Input: part model. Units: mm. Frame: model coordinates. A direction names the side the tool comes from. Round coordinates to 2 decimals unless told otherwise and drop trailing zeros. Write each loop counter-clockwise with the first axis right and the second up, starting at its lowest first coordinate (ties: lowest second). Pieces come first, ordered by that corner, then holes. Notation, with made-up numbers: M -21,14.25 L -3,14.25 A20 cw -3,41.25 Z; hole C -16,84.5 d11. An arc over 180 degrees is marked long. Write each question's results on one line, items separated by ' | '. Start each with the question number.
Autodesk Inventor part; units mm, degrees
ref_plane "YZ Plane" through (0, 0, 0) normal (1, 0, 0) x (0, 1, 0)
ref_plane "XZ Plane" through (0, 0, 0) normal (0, 1, 0) x (-1, 0, 0)
ref_plane "XY Plane" through (0, 0, 0) normal (0, 0, 1) x (1, 0, 0)
sketch "Sketch1" plane through (0, 0, 0) normal (0, 0, 1) x (1, 0, 0)
  line L0 (0, 0) -> (0, 69)
  line L1 (0, 69) -> (70, 69)
  line L2 (70, 69) -> (70, 0)
  line L3 (70, 0) -> (0, 0)
  dimension "d0" = 69
  dimension "d1" = 70
extrude "Extrusion1" add sketch "Sketch1" along normal blind 56
sketch "Sketch2" plane through (0, 0, 56) normal (0, 0, 1) x (1, 0, 0)
  line L0 (0, 0) -> (37, 0)
  line L1 (37, 0) -> (37, 47)
  line L2 (37, 47) -> (0, 47)
  line L3 (0, 47) -> (0, 0)
  dimension "d4" = 37
  dimension "d5" = 47
emboss "Emboss1" sketch "Sketch2" operation cut depth 29 direction (0, 0, -1)
sketch "Sketch3" plane through (0, 0, 56) normal (0, 0, 1) x (1, 0, 0)
  circle A0 centre (62, 61) radius 3
  point P0 (0, 0)
  point P1 (70, 69)
  dimension "d10" = 6
hole "Hole1" at (62, 61, 56) direction (0, 0, -1) diameter 6 end through all
sketch "Sketch4" plane through (0, 0, 0) normal (-1, 0, 0) x (0, 0, 1)
  circle A0 centre (8, 50) radius 3
  point P0 (0, 69)
  dimension "d20" = 6
hole "Hole2" at (0, 50, 8) direction (1, 0, 0) diameter 6 end through all
sketch "Sketch5" plane through (0, 69, 0) normal (0, 1, 0) x (1, 0, 0)
  circle A0 centre (51.2959, -19) radius 3
  dimension "d30" = 6
hole "Hole3" at (51.2959, 69, 19) direction (0, -1, 0) diameter 6 end through all
sketch "Sketch6" plane through (0, 47, 27) normal (0, 0, 1) x (1, 0, 0)
  circle A0 centre (14.5, -32.5) radius 9.5
  dimension "d40" = 19
hole "Hole4" at (14.5, 14.5, 27) direction (0, 0, -1) diameter 19 depth 6
sketch "Sketch7" plane through (37, 0, 56) normal (-1, 0, 0) x (0, 0, 1)
  circle A0 centre (-14.5, 32.5) radius 9.5
  point P0 (-56, 0)
  point P1 (-29, 47)
  dimension "d50" = 19
hole "Hole5" at (37, 32.5, 41.5) direction (1, 0, 0) diameter 19 depth 6
properties part number "Tophjørne1" material "PC/ABS Plastic"
1. Draft query along X for faces 1 (the face through (54.225, 34.017, 18.35)), 2 (the face through (43, 32, 41)), 3 (the face through (11.646, 5.439, 23.958)), 4 (the face through (18, 24, 27)). Return one class per face: +X half, -X half, draft (parallel to the pull), parting line (faces both ways), or undercut.
2. Cut plane D-D on y = 33.5. Output: boundary loops of the cut face in (x, z), and give its area (3 significant figures).
3. Line query: L1, parallel to X at y = 19, z = 19; L2, parallel to Y at x = 49.5, z = 8; L3, parallel to X at y = 14.5, z = 22.65. Output: solid intervals per line, ascending. Write a range as from..to.
4. Cut plane C-C on x = 14.5. Output: boundary loops of the cut face in (y, z).
5. Cut plane B-B on z = 8. Output: boundary loops of the cut face in (x, y), and give its area (3 significant figures).
6. Access query for faces 5 (the face through (18, 47, 42)), 6 (the face through (14, 15, 21)), 7 (the face through (40.042, 29.646, 50.561)). Directions: +Z, -Z, +X, -X, +Y, -Y. A direction counts if a zero-diameter tool reaches every point of the face in a straight line with its end or side. Return the directions, or none.
7. Contact query for flat-ended pins moving along their axis: P1, Ø1.5, axis at x = 33, z = 31, coming from the -Y side; P2, Ø15, axis at x = 16.5, y = 11, coming from the +Z side; P3, Ø9.5, axis at y = 35, z = 45, coming from the -X side. Output: stop coordinate, or through.
8. Cut plane A-A on x = 62. Output: boundary loops of the cut face in (y, z), and give its area (3 significant figures).
Answers follow:
1) face 1: undercut | face 2: -X half | face 3: undercut | face 4: draft
2) outline: M 0,0 L 70,0 L 70,56 L 37,56 L 37,50.95 L 43,50.95 L 43,32.05 L 37,32.05 L 37,27 L 0,27 Z; hole C 51.3,19 d6 | area: 2,710 mm2
3) L1: x = 0..48.3, 54.3..70 | L2: y = 0..47, 53..69 | L3: x = 0..5, 24..70
4) outline: M 0,0 L 69,0 L 69,56 L 47,56 L 47,27 L 24,27 L 24,21 L 5,21 L 5,27 L 0,27 Z; hole C 50,8 d6
5) outline: M 0,0 L 70,0 L 70,47 L 0,47 Z; M 0,53 L 70,53 L 70,69 L 0,69 Z; hole C 62,61 d6 | area: 4,380 mm2
6) face 5: +Z, -X, -Y | face 6: +Z | face 7: -X
7) P1: stops at y = 47 | P2: stops at z = 27 | P3: stops at x = 43
8) outline: M 0,0 L 58,0 L 58,56 L 0,56 Z; M 64,0 L 69,0 L 69,56 L 64,56 Z; hole C 50,8 d6 | area: 3,500 mm2
